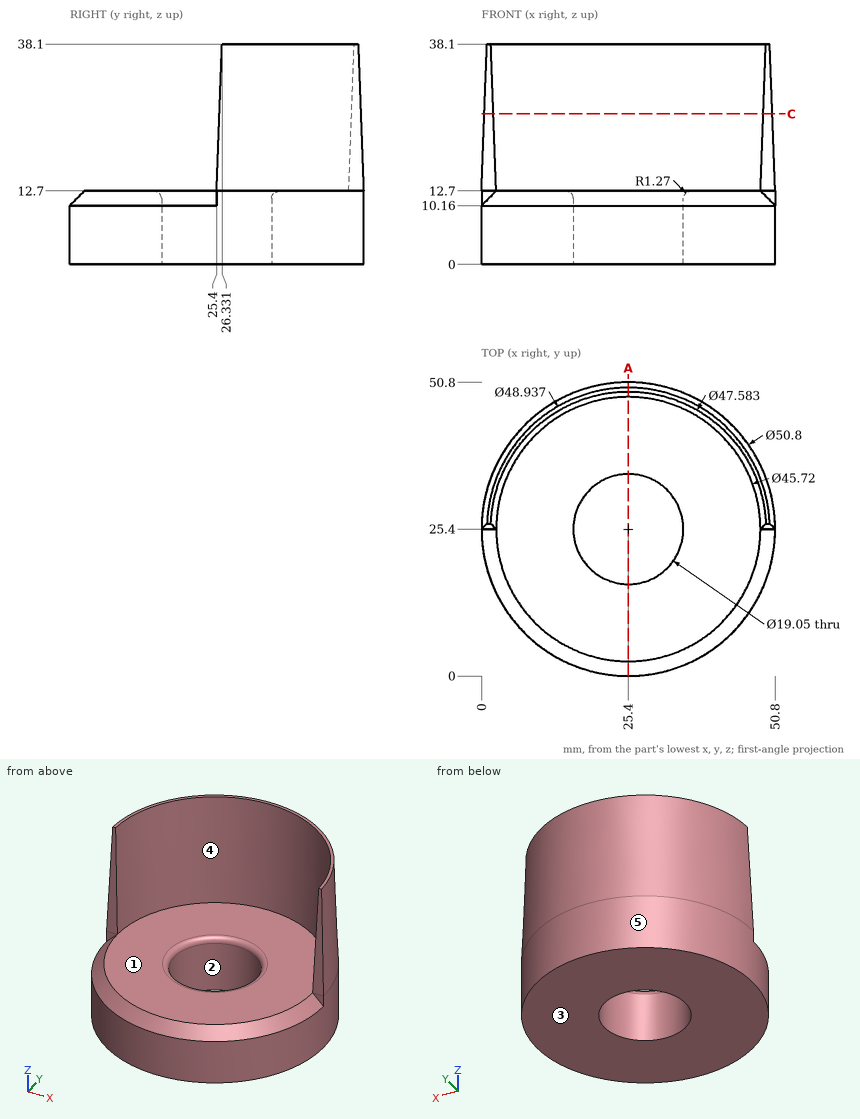
Check sheet for the drawn part. Datum: minimum x, y, z corner. Units: mm. A direction names the side the tool comes from. Round coordinates to 2 decimals unless told otherwise and drop trailing zeros. Loops run counter-clockwise (first coordinate to the right, second up) from the corner with the lowest first, then second, coordinate; pieces in that order, holes last. Notation, with made-up numbers: (79, -30) - (121, -30) arc R27 ccw to (121, -7) - close; hole circle Ø3 at (81, 76.5). An arc over 180 degrees is marked (long way). Answer as a JSON object with one key per item and string values. Group by question number.
Q1. Mould release check, pull along X, two halves, no side actions. Record for the marked faces 3, 4 and 5: released by +X, released by -X, zero draft, split by the parting line, or undercut.
Q2. Sectioned sample at C-C, the plane z = 26. Enter the section's corners in (x, y) (1 decimal), plus the area to 3 significant figures.
Q3. Scan lines: line 1 along X through (y, z) = (25, 8); line 2 along Y through (x, z) = (25.4, 5.75) (1 decimal); line 3 along Z through (x, y) = (35, 11). Record each from-to range of solid material in increasing order. Write a range as [from, to].
Q4. Sectioned sample at A-A, the plane x = 25.4. Enter the section's corners in (y, z) (1 decimal).
Q5. Set-up check for the marked faces 1 and 2: record each of +Z, -Z, +X, -X, +Y, -Y from which the full face is reachable in a straight line by a thin tool's end or side.
Q6. Gauge pin test, flat ends, axial feed: P1, Ø3, axis at y = 25, z = 9, coming from the -X side; P2, Ø4, axis at x = 41.5, z = 22.5, coming from the -Y side; P3, Ø1, axis at y = 21, z = 9.5, coming from the +X side; P4, Ø1, axis at x = 31, z = 17.5, coming from the -Y side. Record the tip position at first contact, or that the pin passes through.
Solution:
{
 "1": {"face 3": "zero draft", "face 4": "undercut", "face 5": "split by the parting line"},
 "2": {"outline": "(0.5, 25.9) - (2.1, 25.9) arc R23.3 cw to (48.7, 25.9) - (50.3, 25.9) arc R24.9 ccw to start", "area": "117 mm²"},
 "3": {"line 1": "x = [0, 15.88], [34.92, 50.8]", "line 2": "y = [0, 15.9], [34.9, 50.8]", "line 3": "z = [0, 12.7]"},
 "4": {"outline": "(0, 0) - (15.9, 0) - (15.9, 11.4) arc R1.3 ccw to (14.6, 12.7) - (2.5, 12.7) - (0, 10.2) - close; (34.9, 0) - (50.8, 0) - (50.8, 12.7) - (49.9, 38.1) - (49.2, 38.1) - (48.3, 12.7) - (36.2, 12.7) arc R1.3 ccw to (34.9, 11.4) - close"},
 "5": {"face 1": "+Z, -Y", "face 2": "+Z, -Z"},
 "6": {"P1": "stops at x = 0", "P2": "stops at y = 39.94", "P3": "stops at x = 50.5", "P4": "stops at y = 47.61"}
}
